Verification items for this drawing (mm, ordinates from the low corner). A direction names the side the tool comes from. Round coordinates to 2 decimals unless told otherwise and drop trailing zeros. Write each loop counter-clockwise with the first axis right and the second up, starting at its lowest first coordinate (ties: lowest second). Pieces come first, ordered by that corner, then holes. Notation, with made-up numbers: (-2.75, 47.25) - (24.25, 47.25) arc R25 cw to (24.25, 62.25) - close; hole circle Ø4 at (78, 2). An arc over 180 degrees is marked (long way). One line per question, with ' | ' between items. Start each with the question number.
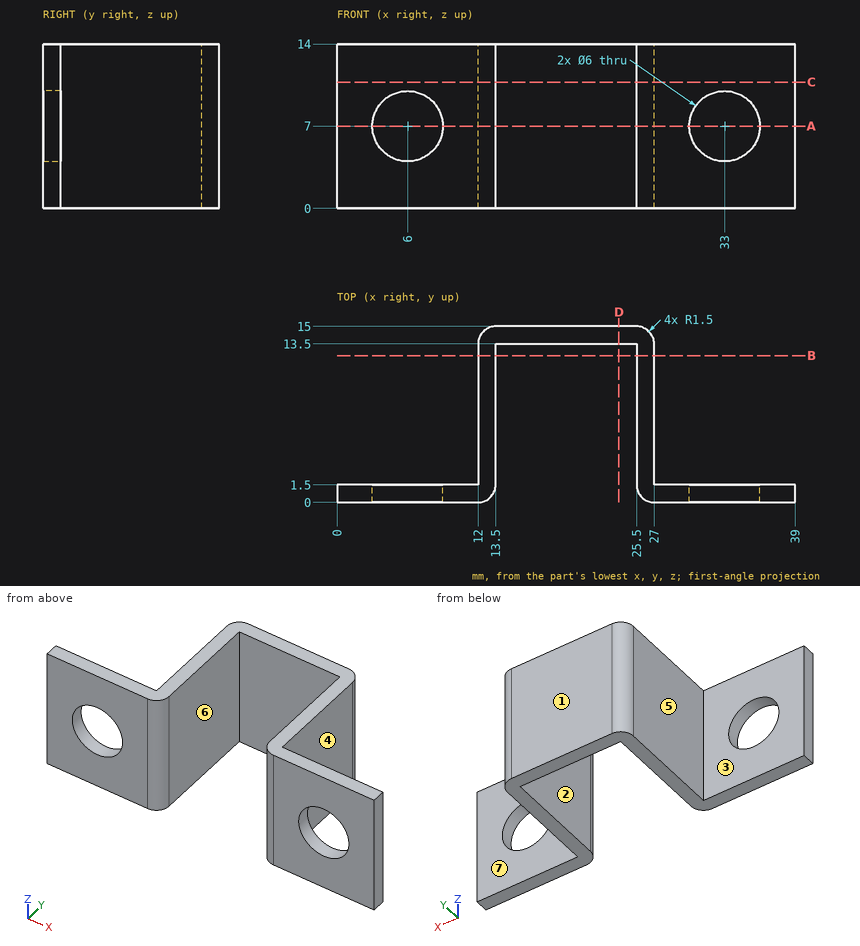
Q1. Section check D-D, the plane x = 24. Record the cut outline in (y, z).
Q2. Section check A-A, the plane z = 7. Record the cut outline in (x, y).
Q3. Set-up check for the marked faces 1, 2, 3 and 4: record each of +Z, -Z, +X, -X, +Y, -Y from which the full face is reachable in a straight line by a thin tool's end or side.
Q4. Thickness scan on line 1 (X direction, y = 5.5, z = 5.5); line 2 (X direction, y = 1.25, z = 7); line 3 (X direction, y = 0.75, z = 7). Record the ranges inside material, lowest first.
Q5. Section check C-C, the plane z = 10.75. Record the cut outline in (x, y).
Q6. Go/stop test with flat-tipped pins: P1, Ø1.5, axis at x = 24, z = 7, coming from the -Y side; P2, Ø6, axis at x = 8.5, z = 6, coming from the +Y side; P3, Ø6, axis at y = 10, z = 4, coming from the +X side. Record where each tip stops, or that it passes through.
Q7. Draft check along X on the marked faces 5, 6 and 7. Enter one of: pulls with the +X half, pulls with the -X half, needs draft (parallel to the pull), parting line crosses it, or undercut.
Q8. Section check B-B, the plane y = 12.5. Record the cut outline in (x, z).
Result sheet:
1) outline: (13.5, 0) - (15, 0) - (15, 14) - (13.5, 14) - close
2) outline: (0, 0) - (3, 0) - (3, 1.5) - (0, 1.5) - close; (9, 0) - (12, 0) arc R1.5 ccw to (13.5, 1.5) - (13.5, 13.5) - (25.5, 13.5) - (25.5, 1.5) arc R1.5 ccw to (27, 0) - (30, 0) - (30, 1.5) - (27, 1.5) - (27, 13.5) arc R1.5 ccw to (25.5, 15) - (13.5, 15) arc R1.5 ccw to (12, 13.5) - (12, 1.5) - (9, 1.5) - close; (36, 0) - (39, 0) - (39, 1.5) - (36, 1.5) - close
3) face 1: +Z, -Z, +X, -X, +Y | face 2: +Z, -Z, -Y | face 3: +Z, -Z, -X, +Y | face 4: +Z, -Z, +X, +Y
4) line 1: 12 to 13.5, 25.5 to 27 | line 2: 0 to 3, 9 to 13.48, 25.52 to 30, 36 to 39 | line 3: 0 to 3, 9 to 13.3, 25.7 to 30, 36 to 39
5) outline: (0, 0) - (12, 0) arc R1.5 ccw to (13.5, 1.5) - (13.5, 13.5) - (25.5, 13.5) - (25.5, 1.5) arc R1.5 ccw to (27, 0) - (39, 0) - (39, 1.5) - (27, 1.5) - (27, 13.5) arc R1.5 ccw to (25.5, 15) - (13.5, 15) arc R1.5 ccw to (12, 13.5) - (12, 1.5) - (0, 1.5) - close
6) P1: y = 13.5 | P2: y = 1.5 | P3: x = 27
7) face 5: pulls with the -X half | face 6: undercut | face 7: needs draft
8) outline: (12, 0) - (13.5, 0) - (13.5, 14) - (12, 14) - close; (25.5, 0) - (27, 0) - (27, 14) - (25.5, 14) - close
